The model under review builds one solid part; all positions refer to its coordinate system, in mm. A direction names the side the tool comes from. Coordinates: 2 decimals unless noted, no trailing zeros. Write each loop counter-clockwise with the first axis right and the second up, starting at its lowest first coordinate (ties: lowest second). Pieces come first, ordered by that corner, then holes. Notation, with made-up numbers: (55, 49.5) -> (81, 49.5) arc R6 cw to (81, 58.5) -> close; hole circle Ø8 at (64.5, 30.5). An arc over 180 degrees is marked (long way). Write each question's results on one line, items separated by ' | '.
```python
from build123d import *

# Parameters (mm, degrees)
F1_DEPTH       = 8
F2_D           = 5
F2_CSINK_D     = 10
F2_CSINK_ANGLE = 90
F3_D           = 12
F4_R           = 2.5


with BuildPart() as f1:
    # F0 (on Front) → F1 (new body)
    with BuildSketch(Plane.XZ):
        Polygon((29, 11.876001), (3, 24), (-29, 24), (-29, -2), (-47.460192, -24), (3, -24), (29, -24), align=None)
    extrude(amount=-F1_DEPTH)

    # F2 (through all)
    with Locations(Plane.XZ):
        with Locations((8, -18), (8, 12)):
            CounterSinkHole(F2_D / 2, F2_CSINK_D / 2, counter_sink_angle=F2_CSINK_ANGLE)

    # F3 (through all)
    with Locations(Plane.XZ):
        with Locations((16, -4)):
            Hole(F3_D / 2)

    # F4
    f4_edges = [f1.edges().sort_by_distance(p)[0] for p in [
        (-47.460192, 4, -24),
        (-29, 4, 24),
        (3, 4, 24),
        (29, 4, 11.876001),
        (29, 4, -24),
    ]]
    fillet(f4_edges, radius=F4_R)


solid = f1.part
```
Q1. Add section A-A (y = 3.25). Write out the cut boundary in (x, z), plus the area to 3 significant figures.
Solution:
outline: (-44.01, -19.89) arc R2.5 ccw to (-42.1, -24) -> (26.5, -24) arc R2.5 ccw to (29, -21.5) -> (29, 10.28) arc R2.5 ccw to (27.56, 12.55) -> (3.5, 23.77) arc R2.5 ccw to (2.45, 24) -> (-26.5, 24) arc R2.5 ccw to (-29, 21.5) -> (-29, -2) -> close; hole circle Ø5 at (8, -18); hole circle Ø5 at (8, 12); hole circle Ø12 at (16, -4) | area: 2,670 mm²
Q2. Add section B-B (x = 17). Write out the cut boundary in (y, z).
Solution:
outline: (0, -24) -> (8, -24) -> (8, -9.92) -> (0, -9.92) -> close; (0, 1.92) -> (8, 1.92) -> (8, 17.47) -> (0, 17.47) -> close
Q3. Add section C-C (z = -4). Write out the cut boundary in (x, y).
Solution:
outline: (-30.68, 0) -> (10, 0) -> (10, 8) -> (-30.68, 8) -> close; (22, 0) -> (29, 0) -> (29, 8) -> (22, 8) -> close
Q4. Add section D-D (x = 8). Write out the cut boundary in (y, z).
Solution:
outline: (0, -24) -> (8, -24) -> (8, -20.5) -> (2.5, -20.5) -> (0, -23) -> close; (0, -13) -> (2.5, -15.5) -> (8, -15.5) -> (8, 9.5) -> (2.5, 9.5) -> (0, 7) -> close; (0, 17) -> (2.5, 14.5) -> (8, 14.5) -> (8, 21.67) -> (0, 21.67) -> close
Q5. Machinability: for faces 1 (the flat face through (-29, 4, 10)), 2 (the flat face through (-8, 8, 0)), which of the approach directions +Z, -Z, +X, -X, +Y, -Y give a long, thin tool a straight path to every point of the face, cutting with its end or side? Answer none if there is none.
Solution:
face 1: +Z, -X, +Y, -Y | face 2: +Z, -Z, +X, -X, +Y
Q6. For line 1 (Z direction, x = 8, y = 5); line 2 (Z direction, x = 6.5, y = 7.5); line 3 (X direction, y = 6.5, z = 7.5), list the stretches that pass through material, from the lowest coordinate up. Write a range as from..to.
Solution:
line 1: -24..-20.5, -15.5..9.5, 14.5..21.67 | line 2: -24..-20, -16..10, 14..22.37 | line 3: -29..29
Q7. Clearance check with flat-ended pins moving along their axes: P1, Ø8, axis at x = 9.5, z = -12, coming from the -Y side; P2, Ø6, axis at x = 8, z = -18, coming from the -Y side; P3, Ø2, axis at x = 13, y = 1.5, coming from the +Z side. State where each tip first meets the part, or that it passes through.
Solution:
P1: y = 0 | P2: y = 2 | P3: z = 19.8
